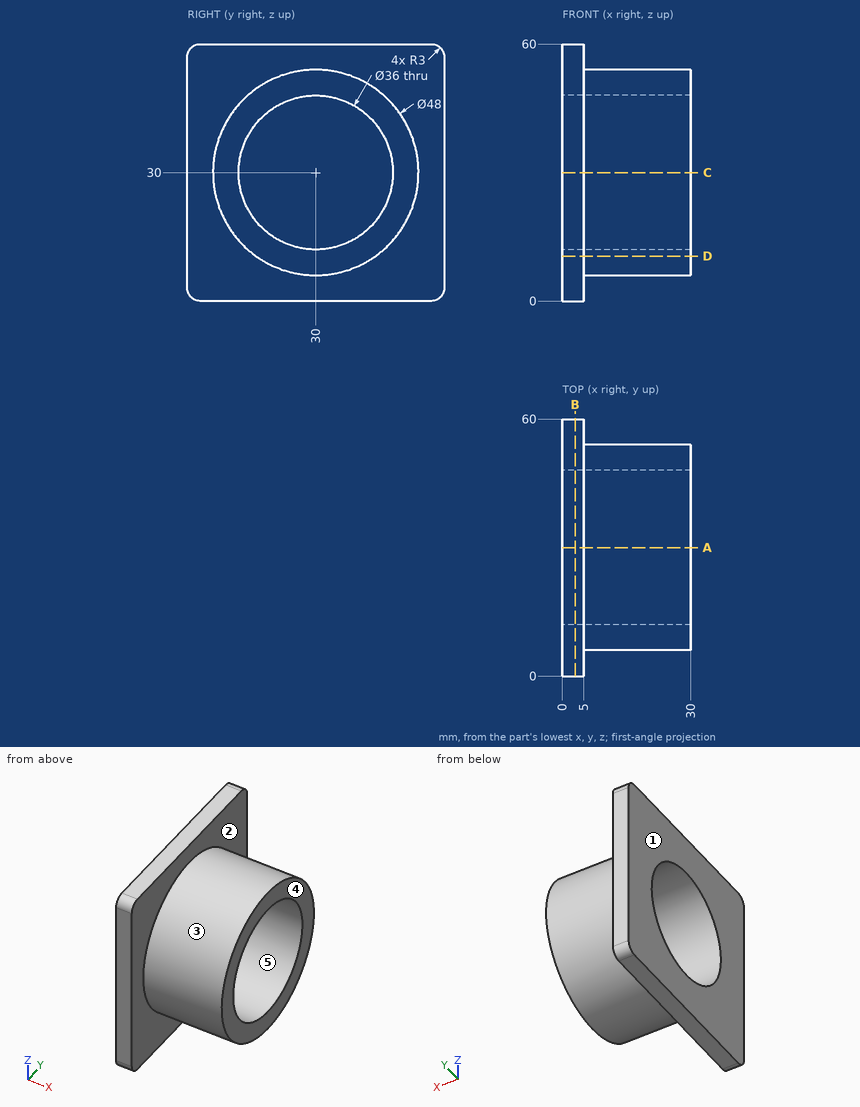
Job drawing, mm, ordinate dimensions from the low corner. One solid piece. A direction names the side the tool comes from. Coordinates: 2 decimals unless noted, no trailing zeros. Order: outer loops, then holes, each group sorted by start corner. A loop starts at its lowest first (then second) coordinate and runs counter-clockwise, first axis right, second up. Notation, with made-up numbers: (48, 48) -> (84, 48) arc R19 ccw to (84, 75) -> close; hole circle Ø11 at (43.5, 45). An arc over 180 degrees is marked (long way). Answer in a Markdown table with one row per item. Add a question column.
Q1. Band-saw the part on B-B, the plane x = 3. List the corners of the cut face in (y, z).
Q2. Drop flat-ended pins along their axis: pin 1 (6 mm diameter, centred on x = 21, y = 15, fed in from -Z); pin 2 (5 mm diameter, centred on x = 11, z = 25, fed in from -Y); pin 3 (4 mm diameter, centred on x = 22, z = 37.5, fed in from -Y); pin 4 (12 mm diameter, centred on y = 25.5, z = 43, fed in from -X). Give the stop position or say it passes through.
Q3. Wall check: line 1 along Y through (x, z) = (18, 30); line 2 along X through (y, z) = (54, 25); line 3 along Y through (x, z) = (16, 18.5). Give the ranges that are in metal, low to high. Write a range as [from, to].
Q4. Which spindle directions (+Z, -Z, +X, -X, +Y, -Y) get a long thin tool onto all of the face, cutting with end or side? Do the marked faces 1 and 2. Say none if no direction does.
Q5. Band-saw the part on D-D, the plane z = 10.5. List the corners of the cut face in (x, y), then the cut area to 4 significant figures.
Q6. Mould opens along Z. For the marked faces 3, 4 and 5 say: +Z half, -Z half, draft (parallel to the pull), parting line (faces both ways), or undercut.
Q7. Band-saw the part on A-A, the plane y = 30. List the corners of the cut face in (x, z).
Answers follow:
| question | item | result |
|---|---|---|
| 1 | outline | (0, 3) arc R3 ccw to (3, 0) -> (57, 0) arc R3 ccw to (60, 3) -> (60, 57) arc R3 ccw to (57, 60) -> (3, 60) arc R3 ccw to (0, 57) -> close; hole circle Ø36 at (30, 30) |
| 2 | pin 1 | z = 9.22 |
| 2 | pin 2 | y = 6.13 |
| 2 | pin 3 | y = 6.64 |
| 2 | pin 4 | x = 0 |
| 3 | line 1 | [6, 12], [48, 54] |
| 3 | line 2 | [0, 5] |
| 3 | line 3 | [8.93, 16.15], [43.85, 51.07] |
| 4 | face 1 | +Z, -Z, -X, +Y, -Y |
| 4 | face 2 | +X |
| 5 | outline | (0, 0) -> (5, 0) -> (5, 16.01) -> (30, 16.01) -> (30, 43.99) -> (5, 43.99) -> (5, 60) -> (0, 60) -> close |
| 5 | area | 1,000 mm^2 |
| 6 | face 3 | parting line |
| 6 | face 4 | draft |
| 6 | face 5 | undercut |
| 7 | outline | (0, 0) -> (5, 0) -> (5, 6) -> (30, 6) -> (30, 12) -> (0, 12) -> close; (0, 48) -> (30, 48) -> (30, 54) -> (5, 54) -> (5, 60) -> (0, 60) -> close |
